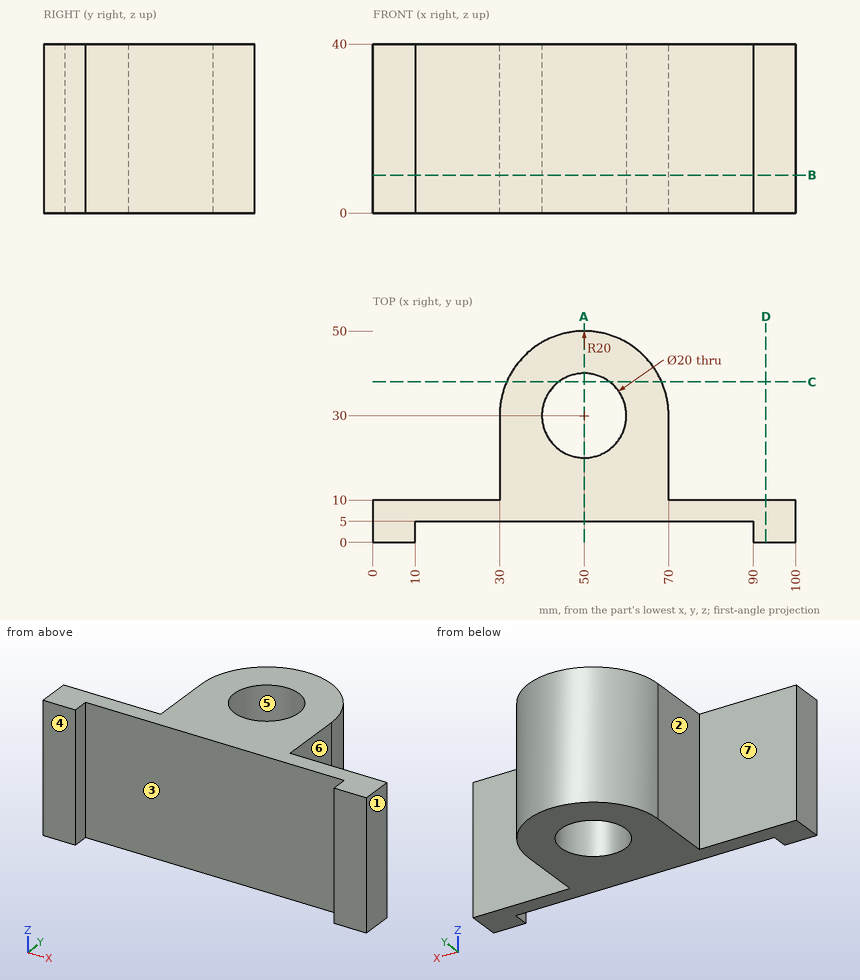
Study the drawing (mm; zero at the part's minimum x, y, z) and answer. A direction names the side the tool comes from. Round coordinates to 2 decimals unless told otherwise and drop trailing zeros. Loops run counter-clockwise (first coordinate to the right, second up) from the corner with the lowest first, then second, coordinate; pieces in that order, holes last. Notation, with made-up numbers: M 11,13.5 L 63,13.5 A27 cw 63,45.5 Z; hole C -21.5,-4.75 d7. An arc over 180 degrees is marked long. One line per question, with ' | ' between items.
Q1. A tool of negligible diameter and unlimited length cuts with its end or side. For the marked faces 5, 6 and 7, from which of +Z, -Z, +X, -X, +Y, -Y can it reach the whole face along a straight path? Write none if from no direction.
Conclusion:
face 5: +Z, -Z | face 6: +Z, -Z, +X, +Y | face 7: +Z, -Z, -X, +Y
Q2. The mould has two halves that part along X. Classify the marked faces 1, 2, 3 and 4: +X half, -X half, draft (parallel to the pull), parting line (faces both ways), or undercut.
Conclusion:
face 1: +X half | face 2: -X half | face 3: undercut | face 4: draft
Q3. Consider line 1 along Y through (x, z) = (50, 15); line 2 along Y through (x, z) = (86, 5.5); line 3 along Y through (x, z) = (96, 29). Determine where each line is inside the solid, lowest interval first. Write a range as from..to.
Conclusion:
line 1: y = 5..20, 40..50 | line 2: y = 5..10 | line 3: y = 0..10
Q4. Find section C-C, the plane y = 38. Give the vertices of the cut face in (x, z).
Conclusion:
outline: M 31.67,0 L 44,0 L 44,40 L 31.67,40 Z; M 56,0 L 68.33,0 L 68.33,40 L 56,40 Z
Q5. Find section D-D, the plane x = 93. Give the vertices of the cut face in (y, z), then the cut area to 3 significant figures.
Conclusion:
outline: M 0,0 L 10,0 L 10,40 L 0,40 Z | area: 400 mm2
Q6. Find section B-B, the plane z = 9. Give the vertices of the cut face in (x, y).
Conclusion:
outline: M 0,0 L 10,0 L 10,5 L 90,5 L 90,0 L 100,0 L 100,10 L 70,10 L 70,30 A20 ccw 30,30 L 30,10 L 0,10 Z; hole C 50,30 d20
Q7. Each of these flat-tipped pins is pushed along its axis until it touches: pin 1 Ø1.5 at (x, z) = (16.5, 20) entering from -Y; pin 2 Ø9 at (x, z) = (11, 14) entering from +Y; pin 3 Ø10 at (y, z) = (24, 14.5) entering from -X. Where does it stop, or does it pass through?
Conclusion:
pin 1: stops at y = 5 | pin 2: stops at y = 10 | pin 3: stops at x = 30
Q8. Find section A-A, the plane x = 50. Give the vertices of the cut face in (y, z).
Conclusion:
outline: M 5,0 L 20,0 L 20,40 L 5,40 Z; M 40,0 L 50,0 L 50,40 L 40,40 Z
